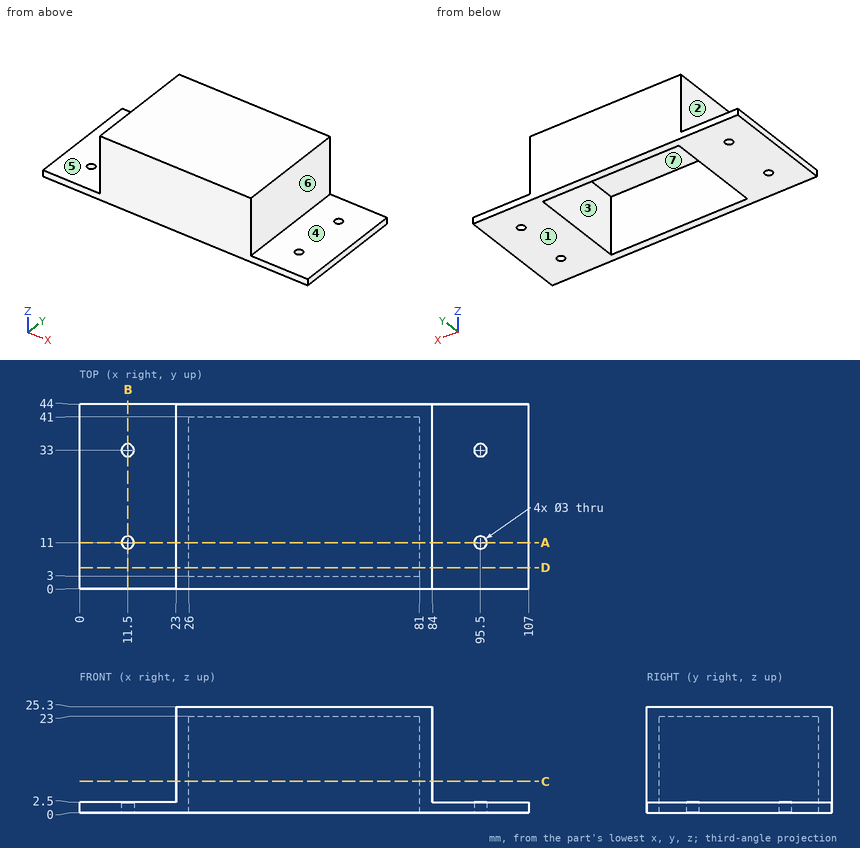
Drawing for the job (mm, zero at the part's lowest x, y, z). A direction names the side the tool comes from. Round coordinates to 2 decimals unless told otherwise and drop trailing zeros. Loops run counter-clockwise (first coordinate to the right, second up) from the corner with the lowest first, then second, coordinate; pieces in that order, holes last.
1. Drop flat-ended pins along their axis: P1, Ø7, axis at y = 32.5, z = 16.5, coming from the +X side; P2, Ø5, axis at x = 95.5, y = 33, coming from the -Z side; P3, Ø1.5, axis at x = 86.5, y = 20, coming from the +Z side; P4, Ø2.5, axis at x = 11.5, y = 11, coming from the -Z side. Give the stop position or say it passes through.
Check values:
P1: stops at x = 84
P2: stops at z = 0
P3: stops at z = 2.5
P4: passes through
2. Band-saw the part on D-D, the plane y = 5. List the corners of the cut face in (x, z).
Check values:
outline: (0, 0) - (26, 0) - (26, 23) - (81, 23) - (81, 0) - (107, 0) - (107, 2.5) - (84, 2.5) - (84, 25.3) - (23, 25.3) - (23, 2.5) - (0, 2.5) - close
3. Mould opens along X. For the marked faces 5, 6 and 7 say: +X half, -X half, draft (parallel to the pull), parting line (faces both ways), or undercut.
Check values:
face 5: draft
face 6: +X half
face 7: undercut
4. Wall check: probe 1 along Y at (x, z) = (11.5, 0.6); probe 2 along Y at (x, z) = (29, 19.5); probe 3 along X at (y, z) = (10, 19.75). Give the ranges that are in metal, low to high.
Check values:
probe 1: y = 0 to 9.5, 12.5 to 31.5, 34.5 to 44
probe 2: y = 0 to 3, 41 to 44
probe 3: x = 23 to 26, 81 to 84
5. Band-saw the part on B-B, the plane x = 11.5. List the corners of the cut face in (y, z).
Check values:
outline: (0, 0) - (9.5, 0) - (9.5, 2.5) - (0, 2.5) - close; (12.5, 0) - (31.5, 0) - (31.5, 2.5) - (12.5, 2.5) - close; (34.5, 0) - (44, 0) - (44, 2.5) - (34.5, 2.5) - close
6. Band-saw the part on C-C, the plane z = 7.5. List the corners of the cut face in (x, y), and give its area (3 significant figures).
Check values:
outline: (23, 0) - (84, 0) - (84, 44) - (23, 44) - close; hole (26, 3) - (81, 3) - (81, 41) - (26, 41) - close
area: 594 mm2
7. Tool access for the marked faces 1, 2, 3 and 4: list every direction of +Z, -Z, +X, -X, +Y, -Y with a clear straight run to the whole face (end or side of a thin tool).
Check values:
face 1: -Z, +X, -X, +Y, -Y
face 2: +Z, -X, +Y, -Y
face 3: -Z
face 4: +Z, +X, +Y, -Y
8. Band-saw the part on A-A, the plane y = 11. List the corners of the cut face in (x, z).
Check values:
outline: (0, 0) - (10, 0) - (10, 2.5) - (0, 2.5) - close; (13, 0) - (26, 0) - (26, 23) - (81, 23) - (81, 0) - (94, 0) - (94, 2.5) - (84, 2.5) - (84, 25.3) - (23, 25.3) - (23, 2.5) - (13, 2.5) - close; (97, 0) - (107, 0) - (107, 2.5) - (97, 2.5) - close
